```python
from build123d import *

# Parameters (mm, degrees)
SKETCH1_W           = 64.5
SKETCH1_H           = 55.5
BOSS_EXTRUDE1_DEPTH = 2
FILLET1_R           = 2
SKETCH2_R           = 1.375
CUT_EXTRUDE1_DEPTH  = 2
SKETCH3_W           = 15.5
SKETCH3_H           = 3.282744178
SKETCH3_W_2         = 8.679035978
BOSS_EXTRUDE2_DEPTH = 6
SKETCH4_R           = 0.75
CUT_EXTRUDE2_DEPTH  = 3
LPATTERN1_COUNT     = 3
LPATTERN1_PITCH     = 3
LPATTERN1_COL_COUNT = 3
LPATTERN1_COL_PITCH = 3
SKETCH5_R           = 0.75
CUT_EXTRUDE3_DEPTH  = 3
LPATTERN2_COUNT     = 3
LPATTERN2_PITCH     = 3
LPATTERN2_COL_COUNT = 3
LPATTERN2_COL_PITCH = 3
SKETCH6_R           = 0.75
CUT_EXTRUDE4_DEPTH  = 3
LPATTERN3_COUNT     = 2
LPATTERN3_PITCH     = 3.7


with BuildPart() as part:
    # Sketch1 → Boss-Extrude1 (new body)
    with BuildSketch(Plane(origin=(0, 0, 0), x_dir=(1, 0, 0), z_dir=(0, 1, 0))):
        Rectangle(SKETCH1_W, SKETCH1_H)
    extrude(amount=BOSS_EXTRUDE1_DEPTH)

    # Fillet1
    fillet1_edges = [part.edges().sort_by_distance(p)[0] for p in [
        (32.25, 1, 27.75),
        (-32.25, 1, 27.75),
        (-32.25, 1, -27.75),
        (32.25, 1, -27.75),
    ]]
    fillet(fillet1_edges, radius=FILLET1_R)

    # Sketch2 → Cut-Extrude1 (cut)
    with BuildSketch(Plane(origin=(0, 2, 0), x_dir=(1, 0, 0), z_dir=(0, 1, 0))):
        with Locations((-29, 24.5)):
            Circle(SKETCH2_R)
        with Locations((29, 24.5)):
            Circle(SKETCH2_R)
        with Locations((29, -24.5)):
            Circle(SKETCH2_R)
        with Locations((-29, -24.5)):
            Circle(SKETCH2_R)
    extrude(amount=-CUT_EXTRUDE1_DEPTH, mode=Mode.SUBTRACT)

    # Sketch3 → Boss-Extrude2 (add)
    with BuildSketch(Plane(origin=(0, 2, 0), x_dir=(1, 0, 0), z_dir=(0, 1, 0))):
        with Locations((-13.190464122, -24.709786803)):
            Rectangle(SKETCH3_W, SKETCH3_H)
        with Locations((3.403133163, -24.709786803)):
            Rectangle(SKETCH3_W, SKETCH3_H)
        with Locations((20.858312779, -24.709786803)):
            Rectangle(SKETCH3_W_2, SKETCH3_H)
    extrude(amount=BOSS_EXTRUDE2_DEPTH)

    # Sketch4 → Cut-Extrude2 (cut)
    with BuildSketch(Plane(origin=(0, 8, 0), x_dir=(1, 0, 0), z_dir=(0, 1, 0))):
        with Locations((-13.190464122, -24.709786803)):
            Circle(SKETCH4_R)
    cut_extrude2 = extrude(amount=-CUT_EXTRUDE2_DEPTH, mode=Mode.SUBTRACT)

    # LPattern1: Cut-Extrude2 ×3
    with Locations(*[(-i * LPATTERN1_PITCH, 0, 0) for i in range(1, LPATTERN1_COUNT)]):
        add(cut_extrude2, mode=Mode.SUBTRACT)

    # LPattern1 col: Cut-Extrude2 ×3
    with Locations(*[(i * LPATTERN1_COL_PITCH, 0, 0) for i in range(1, LPATTERN1_COL_COUNT)]):
        add(cut_extrude2, mode=Mode.SUBTRACT)

    # Sketch5 → Cut-Extrude3 (cut)
    with BuildSketch(Plane(origin=(0, 8, 0), x_dir=(1, 0, 0), z_dir=(0, 1, 0))):
        with Locations((3.403133163, -24.709786803)):
            Circle(SKETCH5_R)
    cut_extrude3 = extrude(amount=-CUT_EXTRUDE3_DEPTH, mode=Mode.SUBTRACT)

    # LPattern2: Cut-Extrude3 ×3
    with Locations(*[(-i * LPATTERN2_PITCH, 0, 0) for i in range(1, LPATTERN2_COUNT)]):
        add(cut_extrude3, mode=Mode.SUBTRACT)

    # LPattern2 col: Cut-Extrude3 ×3
    with Locations(*[(i * LPATTERN2_COL_PITCH, 0, 0) for i in range(1, LPATTERN2_COL_COUNT)]):
        add(cut_extrude3, mode=Mode.SUBTRACT)

    # Sketch6 → Cut-Extrude4 (cut)
    with BuildSketch(Plane(origin=(0, 8, 0), x_dir=(1, 0, 0), z_dir=(0, 1, 0))):
        with Locations((18.945697915, -24.709786803)):
            Circle(SKETCH6_R)
    cut_extrude4 = extrude(amount=-CUT_EXTRUDE4_DEPTH, mode=Mode.SUBTRACT)

    # LPattern3: Cut-Extrude4 ×2
    with Locations(*[(i * LPATTERN3_PITCH, 0, 0) for i in range(1, LPATTERN3_COUNT)]):
        add(cut_extrude4, mode=Mode.SUBTRACT)


solid = part.part
```
Build history of the part. All positions in model axes, mm. A direction names the side the tool comes from. Give positions to 0.01 mm unless a question says otherwise; leave off trailing zeros. Order: outer loops, then holes, each group sorted by start corner. A loop starts at its lowest first (then second) coordinate and runs counter-clockwise, first axis right, second up. Notation, with made-up numbers: M 32.5,69.5 L 71.5,69.5 A16 ccw 71.5,75.5 Z; hole C -22,26 d7. An arc over 180 degrees is marked long. Write item = value, one per line. Start each with the question number.
(1) Probe L1, parallel to X at y = 1.5, z = -24.5 (3 decimals); L2, parallel to Z at x = 29, y = 1.45 (3 decimals); L3, parallel to X at y = 1.5, z = -24. List the from-to ranges inside material, lowest first. Write a range as [from, to].
(2) Slice it at C-C on y = 6. State how many separate pieces and enclosed holes the cut face has, plus the area to 3 significant figures.
(3) Two-plate mould, pull along Z, no slides. Class faces 5 (the flat face through (3, 5, 25)), 6 (the flat face through (-13, 5, 23.068)), 7 (the flat face through (11.153, 5, 25)): released by +Z, released by -Z, zero draft, split by the parting line, or undercut.
(4) Which spindle directions (+Z, -Z, +X, -X, +Y, -Y) get a long thin tool onto all of the face, cutting with end or side? Do faces 1 (the flat face through (-13, 5, 26.351)), 2 (the flat face through (32.25, 1, 0)), 3 (the cylindrical face through (-16.288, 6.521, 23.966)), 4 (the flat face through (-4.347, 5, 25)). Say none if no direction does.
(5) Slice it at B-B on z = -24.5. Write the cut outline in (x, y) (3 decimals), plus the area to 3 significant figures.
(6) Pin check, flat tips, straight feed: pin 1 Ø0.8 at (x, z) = (9.5, 24.5) entering from +Y; pin 2 Ø1.8 at (x, y) = (21.5, 5) entering from -Z; pin 3 Ø16.5 at (x, z) = (-8.5, 5.5) entering from +Y. Stop position of each tip, or through.
(7) Slice it at A-A on y = 3. Write the cut outline in (x, z).
(8) Slice it at D-D on x = 12.5. Write the cut outline in (y, z), plus the area to 3 significant figures.
Responses:
q1.L1 = [-32.25, -30.375], [-27.625, 27.625], [30.375, 32.25]
q1.L2 = [-27.75, -25.875], [-23.125, 23.125], [25.875, 27.75]
q1.L3 = [-32.25, -30.28], [-27.72, 27.72], [30.28, 32.25]
q2.separate_pieces = 3
q2.enclosed_holes = 12
q2.area = 109 mm2
q3.face_5 = undercut
q3.face_6 = released by -Z
q3.face_7 = zero draft
q4.face_1 = +Z, +X, -X, +Y
q4.face_2 = +Z, -Z, +X, +Y, -Y
q4.face_3 = +Y
q4.face_4 = +Z, -Z, +Y
q5.outline = M -32.25,0 L -30.375,0 L -30.375,2 L -32.25,2 Z; M -27.625,0 L 27.625,0 L 27.625,2 L -27.625,2 Z; M 30.375,0 L 32.25,0 L 32.25,2 L 30.375,2 Z
q5.area = 118 mm2
q6.pin_1 = 5
q6.pin_2 = 23.07
q6.pin_3 = 2
q7.outline = M -20.94,23.07 L -5.44,23.07 L -5.44,26.35 L -20.94,26.35 Z; M -4.35,23.07 L 11.15,23.07 L 11.15,26.35 L -4.35,26.35 Z; M 16.52,23.07 L 25.2,23.07 L 25.2,26.35 L 16.52,26.35 Z
q8.outline = M 0,-27.75 L 2,-27.75 L 2,27.75 L 0,27.75 Z
q8.area = 111 mm2
